```python
from build123d import *

# Parameters (mm, degrees)
SKETCH_1_W          = 50
SKETCH_1_H          = 54
SKETCH_1_W_2        = 20
SKETCH_1_H_2        = 40
EXTRUDE_1_DEPTH     = 2
SKETCH_2_R          = 1.25
CUT_EXTRUDE_1_DEPTH = 2
CHAMFER_1_SIZE      = 15
SKETCH_3_W          = 39
SKETCH_3_H          = 2
EXTRUDE_2_DEPTH     = 10
SKETCH_4_W          = 39
SKETCH_4_H          = 2
EXTRUDE_3_DEPTH     = 10
CHAMFER_2_SIZE      = 5
SKETCH_5_R          = 2
CUT_EXTRUDE_2_DEPTH = 10
SKETCH_6_W          = 1.650327519
SKETCH_6_H          = 3.527213322
SKETCH_6_H_2        = 3.728223566
CUT_EXTRUDE_3_DEPTH = 10
FILLET_2_R          = 5


with BuildPart() as part:
    # Эскиз1 → Бобышка-Вытянуть1 (new body)
    with BuildSketch(Plane(origin=(0, 0, 0), x_dir=(1, 0, 0), z_dir=(0, 1, 0))):
        with Locations((-5.839311735, -33.32864132)):
            Rectangle(SKETCH_1_W, SKETCH_1_H)
        with Locations((-5.839311735, -33.32864132)):
            Rectangle(SKETCH_1_W_2, SKETCH_1_H_2, mode=Mode.SUBTRACT)
    extrude(amount=EXTRUDE_1_DEPTH)

    # Эскиз2 → Вырез-Вытянуть1 (cut)
    with BuildSketch(Plane(origin=(0, 2, 0), x_dir=(1, 0, 0), z_dir=(0, 1, 0))):
        with Locations(Location((-10.919311735, -57.39514132, 0), (0, 0, 270))):
            Circle(SKETCH_2_R)
        with Locations(Location((-0.759311735, -57.39514132, 0), (0, 0, 270))):
            Circle(SKETCH_2_R)
        with Locations(Location((-10.919311735, -9.26214132, 0), (0, 0, 270))):
            Circle(SKETCH_2_R)
        with Locations(Location((-0.759311735, -9.26214132, 0), (0, 0, 270))):
            Circle(SKETCH_2_R)
    extrude(amount=-CUT_EXTRUDE_1_DEPTH, mode=Mode.SUBTRACT)

    # Фаска1
    chamfer_1_edges = [part.edges().sort_by_distance(p)[0] for p in [
        (19.160688265, 1, 60.32864132),
        (-30.839311735, 1, 60.32864132),
    ]]
    chamfer(chamfer_1_edges, length=CHAMFER_1_SIZE)

    # Эскиз3 → Бобышка-Вытянуть2 (add)
    with BuildSketch(Plane(origin=(19.160688265, 0, 0), x_dir=(0, 0, -1), z_dir=(1, 0, 0))):
        with Locations((-25.82864132, 1)):
            Rectangle(SKETCH_3_W, SKETCH_3_H)
    extrude(amount=EXTRUDE_2_DEPTH)

    # Эскиз4 → Бобышка-Вытянуть3 (add)
    with BuildSketch(Plane.ZY.offset(30.839311735)):
        with Locations((25.82864132, 1)):
            Rectangle(SKETCH_4_W, SKETCH_4_H)
    extrude(amount=EXTRUDE_3_DEPTH)

    # Фаска2
    chamfer_2_edges = [part.edges().sort_by_distance(p)[0] for p in [
        (29.160688265, 1, 45.32864132),
        (-40.839311735, 1, 45.32864132),
    ]]
    chamfer(chamfer_2_edges, length=CHAMFER_2_SIZE)

    # Эскиз5 → Вырез-Вытянуть2 (cut)
    with BuildSketch(Plane(origin=(0, 2, 0), x_dir=(1, 0, 0), z_dir=(0, 1, 0))):
        with Locations(Location((22.160688265, -38.32864132, 0), (0, 0, 270))):
            Circle(SKETCH_5_R)
        with Locations(Location((-33.839311735, -38.32864132, 0), (0, 0, 270))):
            Circle(SKETCH_5_R)
        with Locations(Location((-33.839311735, -13.32864132, 0), (0, 0, 270))):
            Circle(SKETCH_5_R)
        with Locations(Location((22.160688265, -13.32864132, 0), (0, 0, 270))):
            Circle(SKETCH_5_R)
    extrude(amount=-CUT_EXTRUDE_2_DEPTH, mode=Mode.SUBTRACT)

    # Эскиз6 → Вырез-Вытянуть3 (cut)
    with BuildSketch(Plane.XZ):
        with Locations((-5.761377028, 55.092247981)):
            Rectangle(SKETCH_6_W, SKETCH_6_H)
        with Locations((-5.761377028, 11.464529537)):
            Rectangle(SKETCH_6_W, SKETCH_6_H_2)
    extrude(amount=-CUT_EXTRUDE_3_DEPTH, mode=Mode.SUBTRACT)

    # Скругление2
    fillet_2_edges = [part.edges().sort_by_distance(p)[0] for p in [
        (29.160688265, 1, 6.32864132),
        (-40.839311735, 1, 6.32864132),
    ]]
    fillet(fillet_2_edges, radius=FILLET_2_R)


solid = part.part
```
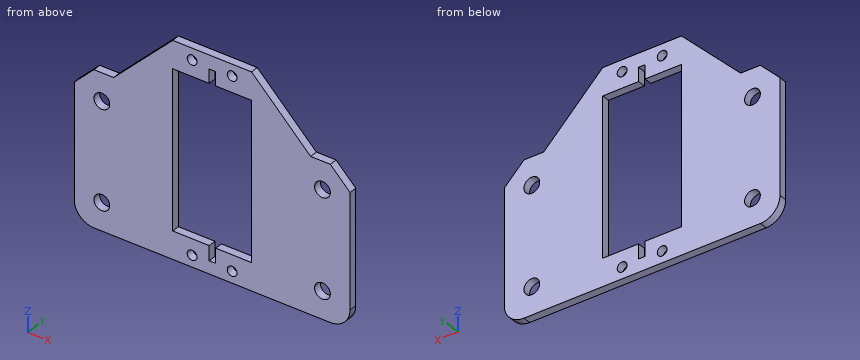
CAD build for the part. Positions are in the model's coordinates, mm. Give positions to 0.01 mm unless a question says otherwise; leave off trailing zeros. Loops run counter-clockwise (first coordinate to the right, second up) from the corner with the lowest first, then second, coordinate; pieces in that order, holes last. Notation, with made-up numbers: (-8.5, -35.5) - (36.5, -35.5) arc R34 cw to (36.5, -2.5) - close; hole circle Ø8 at (72.25, 74). An arc over 180 degrees is marked (long way). Put each result on its own line as item: value.
Q1. Probe line 1 along Z through (x, y) = (-11.5, 1.55); line 2 along X through (y, z) = (1.55, 37.5); line 3 along X through (y, z) = (0.8, 33.5). List the from-to ranges inside material, lowest first.
Filled in:
line 1: z = 6.33 to 8.16, 10.37 to 13.33, 53.33 to 56.29, 58.5 to 60.33
line 2: x = -40.84 to -35.66, -32.02 to -15.84, 4.16 to 20.34, 23.98 to 29.16
line 3: x = -40.84 to -15.84, 4.16 to 29.16
Q2. Slice it at C-C (y = 0.3). Give the number of separate pieces and of enclosed holes in the cut face, plus the area to 3 significant figures.
Filled in:
separate pieces: 1
enclosed holes: 9
area: 2,340 mm²
Q3. Slice it at B-B (x = -13.5). Give the cut face in (y, z).
Filled in:
outline: (0, 6.33) - (2, 6.33) - (2, 13.33) - (0, 13.33) - close; (0, 53.33) - (2, 53.33) - (2, 60.33) - (0, 60.33) - close
Q4. Slice it at A-A (z = 23). Give the cut face in (x, y).
Filled in:
outline: (-40.84, 0) - (-15.84, 0) - (-15.84, 2) - (-40.84, 2) - close; (4.16, 0) - (29.16, 0) - (29.16, 2) - (4.16, 2) - close
Q5. Flat gauge pin, fed straight in: pin 1 (1 mm diameter, centred on y = 1, z = 56, fed in from +X). Where does the tip first touch, or does it go through?
Filled in:
pin 1: stops at x = 8.99
Q6. Slice it at D-D (x = -35). Give the cut face in (y, z), plus the area to 3 significant figures.
Filled in:
outline: (0, 6.33) - (2, 6.33) - (2, 11.7) - (0, 11.7) - close; (0, 14.96) - (2, 14.96) - (2, 36.7) - (0, 36.7) - close; (0, 39.96) - (2, 39.96) - (2, 45.33) - (0, 45.33) - close
area: 65.0 mm²
